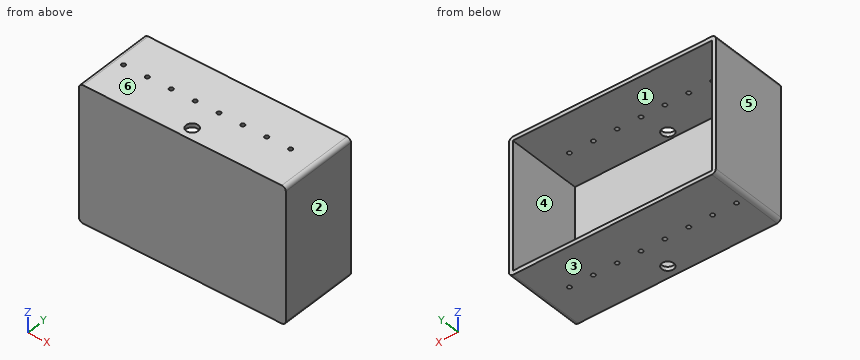
from build123d import *

# Parameters (mm, degrees)
SKETCH1_W           = 160
SKETCH1_H           = 95
BOSS_EXTRUDE1_DEPTH = 130
SKETCH1_3_W         = 160
SKETCH1_3_H         = 95
CUT_EXTRUDE1_DEPTH  = 125
FILLET1_R           = 5
SKETCH2_R           = 2.5
CUT_EXTRUDE2_DEPTH  = 171
SKETCH3_R           = 7.5
CUT_EXTRUDE3_DEPTH  = 171


with BuildPart() as part:
    # Sketch1 → Boss-Extrude1 (new body, symmetric)
    with BuildSketch(Plane(origin=(0, 0, 0), x_dir=(0, 0, -1), z_dir=(1, 0, 0))):
        Polygon((0, 100), (0, 0), (-170, 0), (-170, 100), (-165, 100), (-165, 5), (-5, 5), (-5, 100), align=None)
        with Locations((-85, 52.5)):
            Rectangle(SKETCH1_W, SKETCH1_H)
    extrude(amount=BOSS_EXTRUDE1_DEPTH, both=True)

    # Sketch1_3 → Cut-Extrude1 (cut, symmetric)
    with BuildSketch(Plane(origin=(0, 0, 0), x_dir=(0, 0, -1), z_dir=(1, 0, 0))):
        with Locations((-85, 52.5)):
            Rectangle(SKETCH1_3_W, SKETCH1_3_H)
    extrude(amount=CUT_EXTRUDE1_DEPTH, both=True, mode=Mode.SUBTRACT)

    # Fillet1
    fillet1_edges = [part.edges().sort_by_distance(p)[0] for p in [
        (130, 50, 170),
        (130, 50, 0),
        (-130, 50, 0),
        (-130, 50, 170),
    ]]
    fillet(fillet1_edges, radius=FILLET1_R)

    # Sketch2 → Cut-Extrude2 (cut, through all)
    with BuildSketch(Plane.XY.offset(170)):
        with Locations((95, 50)):
            Circle(SKETCH2_R)
        with Locations((65, 50)):
            Circle(SKETCH2_R)
        with Locations((35, 50)):
            Circle(SKETCH2_R)
        with Locations((5, 50)):
            Circle(SKETCH2_R)
        with Locations((-25, 50)):
            Circle(SKETCH2_R)
        with Locations((-55, 50)):
            Circle(SKETCH2_R)
        with Locations((-85, 50)):
            Circle(SKETCH2_R)
        with Locations((-115, 50)):
            Circle(SKETCH2_R)
    extrude(amount=-CUT_EXTRUDE2_DEPTH, mode=Mode.SUBTRACT)

    # Sketch3 → Cut-Extrude3 (cut, through all)
    with BuildSketch(Plane.XY.offset(170)):
        with Locations((0, 15)):
            Circle(SKETCH3_R)
    extrude(amount=-CUT_EXTRUDE3_DEPTH, mode=Mode.SUBTRACT)


solid = part.part
Build history of the part. All positions in model axes, mm. Face numbers are marked on the shaded views. A direction names the side the tool comes from. Coordinates: 2 decimals unless noted, no trailing zeros. Order: outer loops, then holes, each group sorted by start corner. A loop starts at its lowest first (then second) coordinate and runs counter-clockwise, first axis right, second up. Notation, with made-up numbers: (-39.75, 52) -> (9.25, 52) arc R34 ccw to (9.25, 84) -> close; hole circle Ø6 at (61.25, -25). An arc over 180 degrees is marked (long way). One line per item, written item: value.
(1) Tool access for the marked faces 1 and 2: list every direction of +Z, -Z, +X, -X, +Y, -Y with a clear straight run to the whole face (end or side of a thin tool).
Checked values:
face 1: +Y
face 2: +Z, -Z, +X, +Y, -Y
(2) Mould opens along Z. For the marked faces 3, 4, 5 and 6 say: pulls with the +Z half, pulls with the -Z half, needs draft (parallel to the pull), parting line crosses it, or undercut.
Checked values:
face 3: pulls with the -Z half
face 4: undercut
face 5: needs draft
face 6: pulls with the +Z half
(3) Drop flat-ended pins along their axis: pin 1 Ø12 at (x, z) = (-15, 46.5) entering from +Y; pin 2 Ø4 at (x, y) = (-55, 50) entering from -Z (3 decimals). Give the stop position or say it passes through.
Checked values:
pin 1: y = 5
pin 2: through
(4) Slice it at D-D, the plane z = 156.5. List the corners of the cut face in (x, y), plus the area to 3 significant figures.
Checked values:
outline: (-130, 0) -> (130, 0) -> (130, 100) -> (125, 100) -> (125, 5) -> (-125, 5) -> (-125, 100) -> (-130, 100) -> close
area: 2,250 mm2
(5) Slice it at A-A, the plane x = 55. List the corners of the cut face in (y, z).
Checked values:
outline: (0, 0) -> (100, 0) -> (100, 5) -> (5, 5) -> (5, 165) -> (100, 165) -> (100, 170) -> (0, 170) -> close
(6) Slice it at B-B, the plane y = 15. List the corners of the cut face in (x, z).
Checked values:
outline: (-130, 5) arc R5 ccw to (-125, 0) -> (-7.5, 0) -> (-7.5, 5) -> (-125, 5) -> (-125, 165) -> (-7.5, 165) -> (-7.5, 170) -> (-125, 170) arc R5 ccw to (-130, 165) -> close; (7.5, 0) -> (125, 0) arc R5 ccw to (130, 5) -> (130, 165) arc R5 ccw to (125, 170) -> (7.5, 170) -> (7.5, 165) -> (125, 165) -> (125, 5) -> (7.5, 5) -> close
(7) Slice it at C-C, the plane y = 77.5. List the corners of the cut face in (x, z), plus the area to 3 significant figures.
Checked values:
outline: (-130, 5) arc R5 ccw to (-125, 0) -> (125, 0) arc R5 ccw to (130, 5) -> (130, 165) arc R5 ccw to (125, 170) -> (-125, 170) arc R5 ccw to (-130, 165) -> close; hole (-125, 5) -> (125, 5) -> (125, 165) -> (-125, 165) -> close
area: 4,180 mm2
(8) Probe line 1 (Z direction, x = -9.5, y = 79); line 2 (X direction, y = 16, z = 67); line 3 (Y direction, x = 0, z = 168.2). List the from-to ranges inside material, lowest first. Write a range as [from, to].
Checked values:
line 1: [0, 5], [165, 170]
line 2: [-130, -125], [125, 130]
line 3: [0, 7.5], [22.5, 100]
